Verification items for the finished model (mm, model axes). A direction names the side the tool comes from. Coordinates: 2 decimals unless noted, no trailing zeros. Write each loop counter-clockwise with the first axis right and the second up, starting at its lowest first coordinate (ties: lowest second). Pieces come first, ordered by that corner, then holes. Notation, with made-up numbers: (51.5, 26) - (108.5, 26) arc R15 ccw to (108.5, 51) - close; hole circle Ø7 at (79, 32). An arc over 180 degrees is marked (long way). Use one line per item in the form item = value. Start each with the question number.
(1) Sectioned sample at A-A (z = 7). Record the cut outline in (x, y).
(2) Material ranges on line 1 (X direction, y = -2.5, z = 4); line 2 (X direction, y = 1.75, z = 6); line 3 (Z direction, x = -19, y = 7.75), recorded low to high. Write a range as [from, to].
(3) Sectioned sample at C-C (z = 25). Record the cut outline in (x, y), and give its area (3 significant figures).
(4) Sectioned sample at B-B (x = -9). Record the cut outline in (y, z), and give its area (3 significant figures).
(5) Tool access check on faces 5 (the cylindrical face through (-12.016, 4.721, 28.143)), 6 (the flat face through (0, 12.411, 5)), 7 (the flat face through (-15.972, 0, 20)), 8 (the flat face through (0, -6.592, 12)), 9 (the flat face through (15.972, 0, 20)). Record the directions out of +Z, -Z, +X, -X, +Y, -Y that give a thin tool (end or side, any length) a straight path to the whole face; none if there is none.
(6) Gauge pin test, flat ends, axial feed: pin 1 Ø10 at (x, y) = (-17.5, 9.5) entering from +Z; pin 2 Ø5 at (y, z) = (3.5, 11.5) entering from +X; pin 3 Ø8 at (y, z) = (-2.5, 27) entering from -X; pin 4 Ø1.5 at (y, z) = (-7.5, 21) entering from +X. Record the tip position at first contact, or that the pin passes through.
(7) Sectioned sample at D-D (x = 0). Record the cut outline in (y, z), and give its area (3 significant figures).
(8) Mould release check, pull along X, two halves, no side actions. Record for faces 1 (the cylindrical face through (-12, 0.5, 20.5)), 2 (the cylindrical face through (41.618, -0.273, 4.884)), 3 (the flat face through (7.912, 1.4, 26.4)), 4 (the cylindrical face through (-0.016, -0.092, 12.303)): released by +X, released by -X, zero draft, split by the parting line, or undercut.
from build123d import *

# Parameters (mm, degrees)
F1_DEPTH    = 9.906
F2_W        = 31.9448374212
F2_H        = 13.18457257
F3_DEPTH    = 20.32
F5_DEPTH    = 25.4
F6_T1_DEPTH = 41.6882551367
F6_T3_DEPTH = 41.7866267939
F7_R        = 3.0503938931
F8_DEPTH    = 57.5943291351


# Not quite as in the source:
# - a fillet or chamfer that OpenCascade refuses, or shapes differently, is made with other operations: its cross-section is extruded or revolved along the edge and cut away or added


with BuildPart() as f1:
    # F0 (on Top) → F1 (new body)
    with BuildSketch(Plane.XY):
        with BuildLine():
            Line((-29.21, -12.4109104246), (29.21, -12.4109104246))
            Line((29.21, -12.4109104246), (29.21, -5.0137877216))
            ThreePointArc((29.21, -5.0137877216), (24.1962122784, 0), (29.21, 5.0137877216))
            Line((29.21, 5.0137877216), (29.21, 12.4109104246))
            Line((29.21, 12.4109104246), (-29.21, 12.4109104246))
            Line((-29.21, 12.4109104246), (-29.21, 5.0137877216))
            ThreePointArc((-29.21, 5.0137877216), (-25.6647167027, 3.5452832973), (-24.1962122784, 0))
            ThreePointArc((-24.1962122784, 0), (-25.6647167027, -3.5452832973), (-29.21, -5.0137877216))
            Line((-29.21, -5.0137877216), (-29.21, -12.4109104246))
        make_face()
        with BuildLine():
            ThreePointArc((-29.21, 12.4109104246), (-41.6209104246, 0), (-29.21, -12.4109104246))
            Line((-29.21, -12.4109104246), (-29.21, -5.0137877216))
            ThreePointArc((-29.21, -5.0137877216), (-34.2237877216, 0), (-29.21, 5.0137877216))
            Line((-29.21, 5.0137877216), (-29.21, 12.4109104246))
        make_face()
        with BuildLine():
            Line((29.21, -5.0137877216), (29.21, -12.4109104246))
            ThreePointArc((29.21, -12.4109104246), (41.6209104246, 0), (29.21, 12.4109104246))
            Line((29.21, 12.4109104246), (29.21, 5.0137877216))
            ThreePointArc((29.21, 5.0137877216), (32.7552832973, 3.5452832973), (34.2237877216, 0))
            ThreePointArc((34.2237877216, 0), (32.7552832973, -3.5452832973), (29.21, -5.0137877216))
        make_face()
    extrude(amount=F1_DEPTH)

    # F2 (on face) → F3 (join)
    with BuildSketch(Plane.XY.offset(9.906)):
        Rectangle(F2_W, F2_H)
    extrude(amount=F3_DEPTH)

    # F4 (on face) → F5 (cut)
    with BuildSketch(Plane.XZ.offset(6.592286285)):
        with BuildLine():
            Line((-8.0107270402, 30.226), (-7.9157502647, 20.1440832174))
            ThreePointArc((-7.9157502647, 20.1440832174), (0.1590473721, 12.3041500236), (7.912355383, 20.462159845))
            Line((7.912355383, 20.462159845), (7.912355383, 30.226))
            Line((7.912355383, 30.226), (-8.0107270402, 30.226))
        make_face()
    extrude(amount=-F5_DEPTH, mode=Mode.SUBTRACT)

    # F6: fillet of radius 6.7453126933 on 4 edges, made by hand

    # F6_s2 → F6_t1 (cut)
    with BuildSketch(Plane.YZ.offset(-32.8357004438)):
        with BuildLine():
            ThreePointArc((-6.592286285, 23.4806873067), (-4.6166299384, 28.2503436534), (0.1530264083, 30.226))
            Line((0.1530264083, 30.226), (-6.592286285, 30.226))
            Line((-6.592286285, 30.226), (-6.592286285, 23.4806873067))
        make_face()
        with BuildLine():
            ThreePointArc((6.592286285, 23.4806873067), (4.6166299384, 28.2503436534), (-0.1530264083, 30.226))
            Line((-0.1530264083, 30.226), (6.592286285, 30.226))
            Line((6.592286285, 30.226), (6.592286285, 23.4806873067))
        make_face()
    extrude(amount=F6_T1_DEPTH, mode=Mode.SUBTRACT)

    # F6_s4 → F6_t3 (cut)
    with BuildSketch(Plane.YZ.offset(-8.9509263502)):
        with BuildLine():
            ThreePointArc((-6.592286285, 23.4806873067), (-4.6166299384, 28.2503436534), (0.1530264083, 30.226))
            Line((0.1530264083, 30.226), (-6.592286285, 30.226))
            Line((-6.592286285, 30.226), (-6.592286285, 23.4806873067))
        make_face()
        with BuildLine():
            ThreePointArc((6.592286285, 23.4806873067), (4.6166299384, 28.2503436534), (-0.1530264083, 30.226))
            Line((-0.1530264083, 30.226), (6.592286285, 30.226))
            Line((6.592286285, 30.226), (6.592286285, 23.4806873067))
        make_face()
    extrude(amount=F6_T3_DEPTH, mode=Mode.SUBTRACT)

    # F7 (on face) → F8 (cut, through all)
    with BuildSketch(Plane(origin=(-15.9724187106, 0, 0), x_dir=(0, -1, 0), z_dir=(-1, 0, 0))):
        with Locations((0.1530264083, 23.4806873067)):
            Circle(F7_R)
    extrude(amount=-F8_DEPTH, mode=Mode.SUBTRACT)


solid = f1.part
Answers below:
q1.outline = (-29.21, -12.41) - (29.21, -12.41) arc R12.41 ccw to (29.21, 12.41) - (-29.21, 12.41) arc R12.41 ccw to start; hole circle Ø10.03 at (-29.21, 0); hole circle Ø10.03 at (29.21, 0)
q2.line_1 = [-41.37, -33.56], [-24.86, 24.86], [33.56, 41.37]
q2.line_2 = [-41.5, -33.91], [-24.51, 24.51], [33.91, 41.5]
q2.line_3 = [0, 9.91]
q3.outline = (-15.97, -6.42) - (-7.96, -6.42) - (-7.96, -2.8) - (-15.97, -2.8) - close; (-15.97, 2.49) - (-7.96, 2.49) - (-7.96, 6.42) - (-15.97, 6.42) - close; (7.91, -6.42) - (15.97, -6.42) - (15.97, -2.8) - (7.91, -2.8) - close; (7.91, 2.49) - (15.97, 2.49) - (15.97, 6.42) - (7.91, 6.42) - close
q3.area = 121 mm2
q4.outline = (-12.41, 0) - (12.41, 0) - (12.41, 9.91) - (6.59, 9.91) - (6.59, 23.48) arc R6.75 ccw to (0, 30.22) arc R6.75 ccw to (-6.59, 23.48) - (-6.59, 9.91) - (-12.41, 9.91) - close; hole circle Ø6.1 at (-0.15, 23.48)
q4.area = 465 mm2
q5.face_5 = +Z, +X, -X, +Y
q5.face_6 = +Z, -Z, +X, -X, +Y
q5.face_7 = +Z, -X, +Y, -Y
q5.face_8 = +Z, +X, -X, -Y
q5.face_9 = +Z, +X, +Y, -Y
q6.pin_1 = 28.12
q6.pin_2 = 41.52
q6.pin_3 = -15.97
q6.pin_4 = through
q7.outline = (-12.41, 0) - (12.41, 0) - (12.41, 9.91) - (6.59, 9.91) - (6.59, 12.3) - (-6.59, 12.3) - (-6.59, 9.91) - (-12.41, 9.91) - close
q7.area = 277 mm2
q8.face_1 = zero draft
q8.face_2 = released by +X
q8.face_3 = undercut
q8.face_4 = undercut
